from build123d import *


with BuildPart() as part:
    # Sketch1 → Revolve1 (revolve)
    with BuildSketch(Plane(origin=(0, 0, 0), x_dir=(0, 0, -1), z_dir=(1, 0, 0)), mode=Mode.PRIVATE) as revolve1_sk:
        Polygon((0, 0), (-145.5, 0), (-145.5, 25.7), (-127.3, 25.7), (-125, 28), (-72, 28), (-72, 31), (-56.8, 31), (-54.85, 29.05), (-36, 29.05), (-36, 26.5), (0, 26.5), align=None)
    revolve(revolve1_sk.sketch.rotate(Axis((0, 0, 0), (0, 0, -1)), 90), axis=Axis((0, 0, 0), (0, 0, -1)))

    # Sketch2 → Revolve2 (revolve)
    with BuildSketch(Plane(origin=(0, 0, 0), x_dir=(0, 0, -1), z_dir=(1, 0, 0))):
        Polygon((-62.5, 31), (-62.5, 48), (-57.45, 48), (-57.45, 40), (-58.7, 38.75), (-58.7, 35.25), (-60.55, 35.25), (-60.55, 29), (-62.5, 29), align=None)
    revolve(axis=Axis((0, 48, 62.5), (0, 1, 0)))


solid = part.part
Read the model definition and answer for the solid it produces. Units are mm, in the model's axes. A direction names the side the tool comes from. Coordinates: 2 decimals unless noted, no trailing zeros. Loops run counter-clockwise (first coordinate to the right, second up) from the corner with the lowest first, then second, coordinate; pieces in that order, holes last. Notation, with made-up numbers: (-6.5, 38) -> (4.5, 38) arc R15 ccw to (4.5, 45) -> close; hole circle Ø8 at (58, 31.5). An arc over 180 degrees is marked (long way). Write item = value, one per line. Start each with the question number.
1) Find the intervals of material crossed by L1, parallel to Y at x = -3.5, z = 35; L2, parallel to Y at x = -22.5, z = 93.5; L3, parallel to Z at x = 1.5, y = -27, in increasing order. Write a range as from..to.
2) The part is cut by section A-A, the plane y = 0. Determine the outline of the cut face in (x, z), plus the area to 3 significant figures.
3) For faces 1 (the face through (12.92, 24.84, 98.13)), 2 (the face through (0, 0, 0)), 3 (the face through (-1.141, 36.976, 58.875)), 4 (the face through (-3.45, -26.274, 17.748)), determine the directions among +Z, -Z, +X, -X, +Y, -Y from which every point of the face is accessible in a straight line to the end or side of a thin tool.
4) The part is cut by section C-C, the plane z = 62.5. Determine the outline of the cut face in (x, y), plus the area to 3 significant figures.
5) Given P1, Ø1, axis at y = 21.5, z = 41, coming from the +X side; P2, Ø2, axis at x = -20.5, y = 17.5, coming from the +Z side; P3, Ø5, axis at y = -20, z = 62, coming from the -X side, each flat-ended and moving along its own axis, determine where each tip first touches the part or whether it passes through.
6) The part is cut by section D-D, the plane z = 15.5. Determine the outline of the cut face in (x, y).
7) The mould has two halves that part along Y. Classify faces 5 (the face through (-0.59, 33.06, 60.64)), 6 (the face through (2, 35.25, 61)), 7 (the face through (0, 48, 62)), 8 (the face through (-0.222, 43.944, 67.545)): pulls with the +Y half, pulls with the -Y half, needs draft (parallel to the pull), parting line crosses it, or undercut.
Result:
q1.L1 = -26.27..26.27
q1.L2 = -16.67..16.67
q1.L3 = 36..125.96
q2.outline = (-31, 56.8) -> (-29.05, 54.85) -> (-29.05, 36) -> (-26.5, 36) -> (-26.5, 0) -> (26.5, 0) -> (26.5, 36) -> (29.05, 36) -> (29.05, 54.85) -> (31, 56.8) -> (31, 72) -> (28, 72) -> (28, 125) -> (25.7, 127.3) -> (25.7, 145.5) -> (-25.7, 145.5) -> (-25.7, 127.3) -> (-28, 125) -> (-28, 72) -> (-31, 72) -> close
q2.area = 8,090 mm²
q3.face_1 = +Z
q3.face_2 = -Z, +X, -X, +Y, -Y
q3.face_3 = none
q3.face_4 = -Z
q4.outline = (-5.05, 40) -> (-3.8, 38.75) -> (-3.8, 35.25) -> (-1.95, 35.25) -> (-1.95, 30.94) arc R31 ccw (long way) to (1.95, 30.94) -> (1.95, 35.25) -> (3.8, 35.25) -> (3.8, 38.75) -> (5.05, 40) -> (5.05, 48) -> (-5.05, 48) -> close
q4.area = 3,150 mm²
q5.P1 = 20.07
q5.P2 = 127.05
q5.P3 = -25.59
q6.outline = circle Ø53 at (0, 0)
q7.face_5 = undercut
q7.face_6 = undercut
q7.face_7 = pulls with the +Y half
q7.face_8 = needs draft
